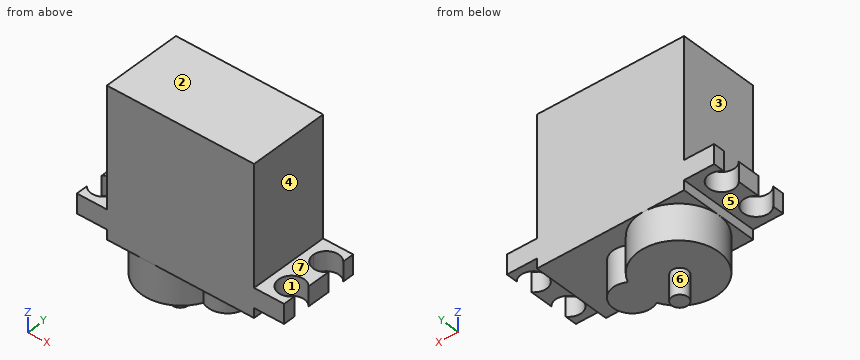
```python
from build123d import *

# Parameters (mm, degrees)
SKETCH1_W             = 11.4
SKETCH1_H             = 12.4
BOSS_EXTRUDE1_DEPTH   = 18.5
SKETCH1_4_W           = 4.65
SKETCH1_4_H           = 12.4
BOSS_EXTRUDE2_DEPTH   = 2.5
BOSS_EXTRUDE2_2_DEPTH = 2.5
SKETCH1_11_W          = 4.65
SKETCH1_11_H          = 12.4
BOSS_EXTRUDE8_DEPTH   = 3
SKETCH1_13_W          = 11.4
SKETCH1_13_H          = 12.4
BOSS_EXTRUDE9_DEPTH   = 4.5
BOSS_EXTRUDE11_DEPTH  = 5.5
SKETCH10_R            = 1.25
BOSS_EXTRUDE12_DEPTH  = 4
BOSS_EXTRUDE13_DEPTH  = 5
SKETCH15_R            = 2
CUT_EXTRUDE1_DEPTH    = 3


with BuildPart() as part:
    # Sketch1 → Boss-Extrude1 (new body)
    with BuildSketch(Plane.XY):
        with Locations((10.35, 6.2)):
            Rectangle(SKETCH1_W, SKETCH1_H)
        with Locations((21.75, 6.2)):
            Rectangle(SKETCH1_W, SKETCH1_H)
    extrude(amount=BOSS_EXTRUDE1_DEPTH)



with BuildPart() as body_2:
    # Sketch1<4> → Boss-Extrude2 (new body)
    with BuildSketch(Plane.XY):
        with Locations((2.325, 6.2)):
            Rectangle(SKETCH1_4_W, SKETCH1_4_H)
    extrude(amount=-BOSS_EXTRUDE2_DEPTH)



with BuildPart() as body_3:
    # Sketch1<4> → Boss-Extrude2 2 (new body)
    with BuildSketch(Plane.XY):
        with Locations((29.775, 6.2)):
            Rectangle(SKETCH1_4_W, SKETCH1_4_H)
    extrude(amount=-BOSS_EXTRUDE2_2_DEPTH)


with BuildPart() as body_2_1:
    add(body_2.part)

    add(body_3.part)  # Boss-Extrude8 merges body 3
    # Sketch1<11> → Boss-Extrude8 (add)
    with BuildSketch(Plane.XY):
        with Locations((29.775, 6.2)):
            Rectangle(SKETCH1_11_W, SKETCH1_11_H)
        with Locations((2.325, 6.2)):
            Rectangle(SKETCH1_11_W, SKETCH1_11_H)
    extrude(amount=-BOSS_EXTRUDE8_DEPTH)


with BuildPart() as part_1:
    add(part.part)

    add(body_2_1.part)  # Boss-Extrude9 merges body 2
    # Sketch1<13> → Boss-Extrude9 (add)
    with BuildSketch(Plane.XY):
        with Locations((21.75, 6.2)):
            Rectangle(SKETCH1_13_W, SKETCH1_13_H)
        with Locations((10.35, 6.2)):
            Rectangle(SKETCH1_13_W, SKETCH1_13_H)
    extrude(amount=-BOSS_EXTRUDE9_DEPTH)

    # Sketch8 → Boss-Extrude11 (add)
    with BuildSketch(Plane(origin=(0, 0, -4.5), x_dir=(-1, 0, 0), z_dir=(0, 0, -1))):
        with BuildLine():
            ThreePointArc((-16.482252321, 3.608140862), (-4.65, 6.2), (-16.482252321, 8.791859138))
            ThreePointArc((-16.482252321, 8.791859138), (-20.992969439, 6.2), (-16.482252321, 3.608140862))
        make_face()
    extrude(amount=BOSS_EXTRUDE11_DEPTH)

    # Sketch10 → Boss-Extrude12 (add)
    with BuildSketch(Plane(origin=(0, 0, -10), x_dir=(-1, 0, 0), z_dir=(0, 0, -1))):
        with Locations((-10.902835345, 5.910258943)):
            Circle(SKETCH10_R)
    extrude(amount=BOSS_EXTRUDE12_DEPTH)

    # Sketch8<2> → Boss-Extrude13 (add)
    with BuildSketch(Plane(origin=(0, 0, -4.5), x_dir=(-1, 0, 0), z_dir=(0, 0, -1))):
        with BuildLine():
            ThreePointArc((-16.482252321, 3.608140862), (-4.65, 6.2), (-16.482252321, 8.791859138))
            ThreePointArc((-16.482252321, 8.791859138), (-20.992969439, 6.2), (-16.482252321, 3.608140862))
        make_face()
    extrude(amount=BOSS_EXTRUDE13_DEPTH)

    # Sketch15 → Cut-Extrude1 (cut)
    with BuildSketch(Plane(origin=(0, 0, -3), x_dir=(-1, 0, 0), z_dir=(0, 0, -1))):
        with BuildLine():
            ThreePointArc((-32.1, 10.629307241), (-32.605696731, 9.3), (-32.1, 7.970692759))
            Line((-32.1, 7.970692759), (-32.1, 10.629307241))
        make_face()
        with BuildLine():
            Line((-32.1, 10.629307241), (-32.1, 7.970692759))
            ThreePointArc((-32.1, 7.970692759), (-29.894573162, 7.430694442), (-28.605696731, 9.3))
            ThreePointArc((-28.605696731, 9.3), (-29.894573162, 11.169305558), (-32.1, 10.629307241))
        make_face()
        with Locations((-1.494303269, 9.3)):
            Circle(SKETCH15_R)
        with BuildLine():
            ThreePointArc((0, 4.429307241), (-3.494303269, 3.1), (0, 1.770692759))
            Line((0, 1.770692759), (0, 4.429307241))
        make_face()
        with BuildLine():
            Line((0, 4.429307241), (0, 1.770692759))
            ThreePointArc((0, 1.770692759), (0.375002289, 2.38887643), (0.505696731, 3.1))
            ThreePointArc((0.505696731, 3.1), (0.375002289, 3.81112357), (0, 4.429307241))
        make_face()
        with Locations((-30.567157508, 3.111527569)):
            Circle(SKETCH15_R)
    extrude(amount=-CUT_EXTRUDE1_DEPTH, mode=Mode.SUBTRACT)


solid = part_1.part
```
Geometry: final body of the model. Coordinates: model frame, mm. Face numbers are marked on the shaded views. A direction names the side the tool comes from. Round coordinates to 2 decimals unless told otherwise and drop trailing zeros. Order: outer loops, then holes, each group sorted by start corner. A loop starts at its lowest first (then second) coordinate and runs counter-clockwise, first axis right, second up. Notation, with made-up numbers: (0, 21.25) -> (43, 21.25) arc R27 ccw to (43, 51.25) -> close; hole circle Ø9 at (-32, 31.25). An arc over 180 degrees is marked (long way). Write each question's results on one line, items separated by ' | '.
Q1. Ray query, line 1 along X through (y, z) = (7.5, 5); line 2 along X through (y, z) = (6, -10.5); line 3 along Z through (x, y) = (23, 11.75). Return the intervals inside material, ascending.
Response values:
line 1: 4.65 to 27.45 | line 2: 9.66 to 12.15 | line 3: -4.5 to 18.5
Q2. Section query B-B (z = 1). Output: boundary loops of the cut face in (x, y).
Response values:
outline: (4.65, 0) -> (27.45, 0) -> (27.45, 12.4) -> (4.65, 12.4) -> close
Q3. Section query C-C (x = 17). Output: boundary loops of the cut face in (y, z).
Response values:
outline: (0, -4.5) -> (3.37, -4.5) -> (3.37, -10) -> (9.03, -10) -> (9.03, -4.5) -> (12.4, -4.5) -> (12.4, 18.5) -> (0, 18.5) -> close
Q4. Access query for the marked faces 5, 6 and 7. Directions: +Z, -Z, +X, -X, +Y, -Y. A direction counts if a zero-diameter tool reaches every point of the face in a straight line with its end or side. Return the directions, or none.
Response values:
face 5: -Z, -X, +Y, -Y | face 6: -Z | face 7: +Z, +X, +Y, -Y
Q5. Pull-direction query (X, two-part tool) for the marked faces 1, 2, 3 and 4; classes: released by +X, released by -X, zero draft, split by the parting line, or undercut.
Response values:
face 1: undercut | face 2: zero draft | face 3: released by -X | face 4: released by +X
Q6. Pin query (flat end, axial travel): pin 1 Ø5 at (x, y) = (1.49, 9.3) entering from +Z; pin 2 Ø3.5 at (x, y) = (30, 5.5) entering from -Z; pin 3 Ø1 at (y, z) = (3, 9) entering from -X. Return the tip coordinate at first contact, or that it passes through.
Response values:
pin 1: z = 0 | pin 2: z = -3 | pin 3: x = 4.65
Q7. Section query A-A (x = 3). Output: boundary loops of the cut face in (y, z).
Response values:
outline: (0, -3) -> (1.78, -3) -> (1.78, 0) -> (0, 0) -> close; (4.42, -3) -> (7.98, -3) -> (7.98, 0) -> (4.42, 0) -> close; (10.62, -3) -> (12.4, -3) -> (12.4, 0) -> (10.62, 0) -> close
Q8. Section query D-D (z = -5). Output: boundary loops of the cut face in (x, y), and give its area (3 significant figures).
Response values:
outline: (16.48, 3.61) arc R3 ccw (long way) to (16.48, 8.79) arc R6.2 ccw (long way) to start | area: 142 mm²
